Build history of the part. All positions in model axes, mm. A direction names the side the tool comes from. Give positions to 0.01 mm unless a question says otherwise; leave off trailing zeros. One line per question, with ' | ' between items. Start each with the question number.
(1) Pull direction Z, two halves, no side cores. Call faces 4 (the flat face through (52, 53, -25)), 5 (the flat face through (81, 53, -52)), 6 (the flat face through (3, -5, -51)), 7 (the flat face through (51, -5, -17)): released by +Z, released by -Z, zero draft, split by the parting line, or undercut.
(2) Drill centre lines: probe 1 along X at (y, z) = (-5, -86); probe 2 along X at (y, z) = (14, -55); probe 3 along Z at (x, y) = (36, 97.5). Where is each one in solid material? Low to high. Write a range as from..to.
(3) Pin check, flat tips, straight feed: P1, Ø1.5, axis at x = 51.5, y = 36.5, coming from the +Z side (3 decimals); P2, Ø18, axis at x = 14, z = -86.5, coming from the -Y side; P3, Ø13.5, axis at x = 93.5, y = 45.5, coming from the +Z side; P4, Ø1.5, axis at y = 29, z = -83, coming from the -X side. Stop position of each tip, or through.
(4) Tool access for faces 1 (the cylindrical face through (80.89, 57.58, -66.83)), 2 (the flat face through (18, 10, -86)), 3 (the flat face through (101, -5, -77)): list every direction of +Z, -Z, +X, -X, +Y, -Y with a clear straight run to the whole face (end or side of a thin tool).
from build123d import *

# Parameters (mm, degrees)
SKETCH1_W           = 104
SKETCH1_H           = 104
BOSS_EXTRUDE1_DEPTH = 57.5
BOSS_EXTRUDE1_TAPER = 23
SKETCH2_R           = 25
CUT_EXTRUDE1_DEPTH  = 187.700294763
FILLET1_R           = 15
SKETCH3_R           = 35
CUT_EXTRUDE2_DEPTH  = 10
CUT_EXTRUDE3_START  = -10
SKETCH4_R           = 35
CUT_EXTRUDE3_DEPTH  = 10
SKETCH5_W           = 52
SKETCH5_H           = 52
CUT_EXTRUDE4_DEPTH  = 187.700294763
BOSS_EXTRUDE2_DEPTH = 10
FILLET2_R           = 5
FILLET3_R           = 5
CUT_EXTRUDE5_DEPTH  = 10


with BuildPart() as part:
    # Sketch1 → Boss-Extrude1 (new body)
    with BuildSketch(Plane(origin=(0, 0, 0), x_dir=(1, 0, 0), z_dir=(0, 1, 0))):
        with Locations((52, 52)):
            Rectangle(SKETCH1_W, SKETCH1_H)
    extrude(amount=BOSS_EXTRUDE1_DEPTH, taper=BOSS_EXTRUDE1_TAPER)

    # Mirror1: part across plane


with BuildPart() as part_1:
    add(part.part)
    add(part.part.mirror(Plane(origin=(0, 57.5, 0), x_dir=(0, 0, 1), z_dir=(0, -1, 0))))

    # Sketch2 → Cut-Extrude1 (cut, through all)
    with BuildSketch(Plane(origin=(0, 115, 0), x_dir=(1, 0, 0), z_dir=(0, 1, 0))):
        with Locations(Location((52, 52, 0), (0, 0, 270))):
            Circle(SKETCH2_R)
    extrude(amount=-CUT_EXTRUDE1_DEPTH, mode=Mode.SUBTRACT)

    # Fillet1
    # the kernel refuses this fillet: 15 mm, written as the material it adds along each edge
    with BuildSketch(Plane(origin=(24.407301932, 57.5, -95.510503676), x_dir=(-0.39073112848927455, -0.9205048534524399, 0), z_dir=(0, 0, 1))) as fillet1_piece_1_section:
        with BuildLine():
            CenterArc((FILLET1_R * 0.42447481621, -FILLET1_R), FILLET1_R, 90, 46)
            Line((-FILLET1_R * 0.294864984129, -FILLET1_R * 0.305341629541), (0, 0))
            Line((0, 0), (FILLET1_R * 0.42447481621, 0))
        make_face()
    fillet1_piece_1 = extrude(amount=87.021007352, mode=Mode.PRIVATE)
    fillet1_piece_1 = fillet1_piece_1 - Plane(origin=(24.407301932, 57.5, -8.111896271), x_dir=(0, -0.39073112848927466, -0.9205048534524399), z_dir=(-1, 0, 0)) * Cylinder(15, 200, mode=Mode.PRIVATE)
    fillet1_piece_1 = fillet1_piece_1 - Plane(origin=(24.407301932, 57.5, -95.888103729), x_dir=(0, -0.3907311284892748, 0.9205048534524398), z_dir=(1, 0, 0)) * Cylinder(15, 200, mode=Mode.PRIVATE)
    add(fillet1_piece_1)
    with BuildSketch(Plane(origin=(8.489496324, 57.5, -24.407301932), x_dir=(0, -0.9205048534524399, 0.39073112848927455), z_dir=(1, 0, 0))) as fillet1_piece_2_section:
        with BuildLine():
            CenterArc((FILLET1_R * 0.42447481621, -FILLET1_R), FILLET1_R, 90, 46)
            Line((-FILLET1_R * 0.294864984129, -FILLET1_R * 0.305341629541), (0, 0))
            Line((0, 0), (FILLET1_R * 0.42447481621, 0))
        make_face()
    fillet1_piece_2 = extrude(amount=87.021007352, mode=Mode.PRIVATE)
    fillet1_piece_2 = fillet1_piece_2 - Plane(origin=(95.888103729, 57.5, -24.407301932), x_dir=(-0.9205048534524398, -0.3907311284892748, 0), z_dir=(0, 0, 1)) * Cylinder(15, 200, mode=Mode.PRIVATE)
    fillet1_piece_2 = fillet1_piece_2 - Plane(origin=(8.111896271, 57.5, -24.407301932), x_dir=(0.9205048534524399, -0.39073112848927466, 0), z_dir=(0, 0, -1)) * Cylinder(15, 200, mode=Mode.PRIVATE)
    add(fillet1_piece_2)
    with BuildSketch(Plane(origin=(79.592698068, 57.5, -8.489496324), x_dir=(0.39073112848927455, -0.9205048534524399, 0), z_dir=(0, 0, -1))) as fillet1_piece_3_section:
        with BuildLine():
            CenterArc((FILLET1_R * 0.42447481621, -FILLET1_R), FILLET1_R, 90, 46)
            Line((-FILLET1_R * 0.294864984129, -FILLET1_R * 0.305341629541), (0, 0))
            Line((0, 0), (FILLET1_R * 0.42447481621, 0))
        make_face()
    fillet1_piece_3 = extrude(amount=87.021007352, mode=Mode.PRIVATE)
    fillet1_piece_3 = fillet1_piece_3 - Plane(origin=(79.592698068, 57.5, -8.111896271), x_dir=(0, -0.39073112848927466, -0.9205048534524399), z_dir=(-1, 0, 0)) * Cylinder(15, 200, mode=Mode.PRIVATE)
    fillet1_piece_3 = fillet1_piece_3 - Plane(origin=(79.592698068, 57.5, -95.888103729), x_dir=(0, -0.3907311284892748, 0.9205048534524398), z_dir=(1, 0, 0)) * Cylinder(15, 200, mode=Mode.PRIVATE)
    add(fillet1_piece_3)
    with BuildSketch(Plane(origin=(95.510503676, 57.5, -79.592698068), x_dir=(0, -0.9205048534524399, -0.39073112848927455), z_dir=(-1, 0, 0))) as fillet1_piece_4_section:
        with BuildLine():
            CenterArc((FILLET1_R * 0.42447481621, -FILLET1_R), FILLET1_R, 90, 46)
            Line((-FILLET1_R * 0.294864984129, -FILLET1_R * 0.305341629541), (0, 0))
            Line((0, 0), (FILLET1_R * 0.42447481621, 0))
        make_face()
    fillet1_piece_4 = extrude(amount=87.021007352, mode=Mode.PRIVATE)
    fillet1_piece_4 = fillet1_piece_4 - Plane(origin=(95.888103729, 57.5, -79.592698068), x_dir=(-0.9205048534524398, -0.3907311284892748, 0), z_dir=(0, 0, 1)) * Cylinder(15, 200, mode=Mode.PRIVATE)
    fillet1_piece_4 = fillet1_piece_4 - Plane(origin=(8.111896271, 57.5, -79.592698068), x_dir=(0.9205048534524399, -0.39073112848927466, 0), z_dir=(0, 0, -1)) * Cylinder(15, 200, mode=Mode.PRIVATE)
    add(fillet1_piece_4)

    # Sketch3 → Cut-Extrude2 (cut)
    with BuildSketch(Plane(origin=(0, 115, 0), x_dir=(1, 0, 0), z_dir=(0, 1, 0))):
        with Locations(Location((52, 52, 0), (0, 0, 270))):
            Circle(SKETCH3_R)
    extrude(amount=-CUT_EXTRUDE2_DEPTH, mode=Mode.SUBTRACT)

    # Sketch4 → Cut-Extrude3 (cut)
    with BuildSketch(Plane.XZ.offset(CUT_EXTRUDE3_START)):
        with Locations(Location((52, -52, 0), (0, 0, 90))):
            Circle(SKETCH4_R)
    extrude(amount=CUT_EXTRUDE3_DEPTH, mode=Mode.SUBTRACT)

    # Sketch5 → Cut-Extrude4 (cut, through all)
    with BuildSketch(Plane(origin=(0, 115, 0), x_dir=(1, 0, 0), z_dir=(0, 1, 0))):
        with Locations((78, 26)):
            Rectangle(SKETCH5_W, SKETCH5_H)
    extrude(amount=-CUT_EXTRUDE4_DEPTH, mode=Mode.SUBTRACT)

    # Sketch7 → Boss-Extrude2 (add)
    with BuildSketch(Plane.XZ):
        Polygon((49, -17), (49, -3), (3, -3), (3, -101), (101, -101), (101, -52), (104, -52), (104, -104), (0, -104), (0, 0), (52, 0), (52, -17), align=None)
    extrude(amount=BOSS_EXTRUDE2_DEPTH)

    # Fillet2
    fillet2_edges = [part_1.edges().sort_by_distance(p)[0] for p in [
        (52, 0, -101),
        (26, 0, 0),
        (0, 0, -52),
        (104, 0, -78),
    ]]
    fillet(fillet2_edges, radius=FILLET2_R)

    # Fillet3
    fillet3_edges = [part_1.edges().sort_by_distance(p)[0] for p in [
        (52, 0, -104),
    ]]
    fillet(fillet3_edges, radius=FILLET3_R)

    # Sketch8 → Cut-Extrude5 (cut)
    with BuildSketch(Plane.XZ):
        with BuildLine():
            Line((14.682837651, -10.358480419), (25.323985369, -20.930423251))
            ThreePointArc((25.323985369, -20.930423251), (25.337826346, -25.173041361), (21.095208236, -25.186882338))
            Line((21.095208236, -25.186882338), (10.454060518, -14.614939506))
            ThreePointArc((10.454060518, -14.614939506), (10.440219541, -10.372321396), (14.682837651, -10.358480419))
        make_face()
        with BuildLine():
            Line((14.682837651, -93.641519581), (25.323985369, -83.069576749))
            ThreePointArc((25.323985369, -83.069576749), (25.337826346, -78.826958639), (21.095208236, -78.813117662))
            Line((21.095208236, -78.813117662), (10.454060518, -89.385060494))
            ThreePointArc((10.454060518, -89.385060494), (10.440219541, -93.627678604), (14.682837651, -93.641519581))
        make_face()
        with BuildLine():
            Line((93.938828765, -88.715537796), (83.246195736, -78.19567093))
            ThreePointArc((83.246195736, -78.19567093), (79.003695757, -78.230224162), (79.038248989, -82.472724142))
            Line((79.038248989, -82.472724142), (89.730882019, -92.992591008))
            ThreePointArc((89.730882019, -92.992591008), (93.973381998, -92.958037776), (93.938828765, -88.715537796))
        make_face()
    extrude(amount=-CUT_EXTRUDE5_DEPTH, mode=Mode.SUBTRACT)


solid = part_1.part
Results:
1) face 4: zero draft | face 5: released by +Z | face 6: undercut | face 7: undercut
2) probe 1: x = 0..3, 101..104 | probe 2: x = 5.94..27.18, 76.82..98.06 | probe 3: z = -96.57..-71.21, -32.79..-7.43
3) P1: stops at z = -15.175 | P2: stops at y = 0 | P3: passes through | P4: stops at x = 11.99
4) face 1: +Z, -Z, +X | face 2: -Y | face 3: +Z, -Y
